For this review, take the finished solid that the model builds, in its own axes (mm). Coordinates: 2 decimals unless noted, no trailing zeros. Write each loop counter-clockwise with the first axis right and the second up, starting at its lowest first coordinate (ties: lowest second). Pieces come first, ordered by that corner, then holes. Notation, with made-up numbers: M 29.25,-34 L 36.25,-34 A25 ccw 36.25,-11 Z; hole C 12.25,53.25 d4. An arc over 180 degrees is marked long. Return JSON: item names as keys, results as strings.
```python
from build123d import *

# Parameters (mm, degrees)
THREAD1_PITCH = 2


with BuildPart() as part:
    # Sketch1 → Revolve3 (revolve)
    with BuildSketch(Plane.XY):
        with BuildLine():
            Line((-5, 97.371710471), (-5, 94.868329805))
            ThreePointArc((-5, 94.868329805), (65.383484153, 68.92024376), (95, 0))
            Line((95, 0), (100, 0))
            ThreePointArc((100, 0), (72.456883731, 68.92024376), (5, 99.874921777))
            Line((5, 99.874921777), (5, 97.371710471))
            Line((5, 97.371710471), (-5, 97.371710471))
        make_face()
    revolve(axis=Axis((-5, 0, 0), (1, 0, 0)))

    # Thread1: arcs per turn and ends read off the stored shape
    # Thread1: the profile of Thread Profile2 profile screwed along a right-hand helix through 5 turns, 10 arcs to a turn; built about Z, then put on its axis
    thread1_z = Axis((0, 0, 0), (0, 0, 1))
    thread1_corners = [(97.371410471, 0, -0.000173205), (98.454242221, 0, 0.624999997), (98.454242221, 0, 0.874999997), (97.371410471, 0, 1.5001732)]
    with BuildLine(mode=Mode.PRIVATE) as thread1_profile:
        Line(thread1_corners[0], thread1_corners[1])
        Line(thread1_corners[1], thread1_corners[2])
        Line(thread1_corners[2], thread1_corners[3])
        Line(thread1_corners[3], thread1_corners[0])
    thread1_cap = Face(thread1_profile.wire())
    thread1_turn_angles = [0, 18, 36, 54, 72, 90, 108, 126, 144, 162, 180, 198, 216, 234, 252, 270, 288, 306, 324, 342, 360]
    thread1_turn_weights = [1, 0.9510565162951535, 1, 0.9510565162951535, 1, 0.9510565162951535, 1, 0.9510565162951535, 1, 0.9510565162951535, 1, 0.9510565162951535, 1, 0.9510565162951535, 1, 0.9510565162951535, 1, 0.9510565162951535, 1, 0.9510565162951535, 1]
    thread1_turn_rails = [Edge.make_bspline([Vector(p[0], p[1], 0).rotate(thread1_z, thread1_turn_angles[k]) / thread1_turn_weights[k] + Vector(0, 0, p[2] + THREAD1_PITCH * thread1_turn_angles[k] / 360) for k in range(21)], [0, 0, 0, 1, 1, 2, 2, 3, 3, 4, 4, 5, 5, 6, 6, 7, 7, 8, 8, 9, 9, 10, 10, 10], 2, thread1_turn_weights) for p in thread1_corners]
    thread1_turn_sides = [Face.make_surface_from_curves(thread1_turn_rails[p[0]], thread1_turn_rails[p[1]]) for p in [(0, 1), (1, 2), (2, 3), (3, 0)]]
    thread1 = Plane(origin=(-5, 0, 0), x_dir=(0, 0, -1), z_dir=(1, 0, 0)) * Solid(Shell([*[p.moved(Location((0, 0, THREAD1_PITCH * i))) for i in range(5) for p in thread1_turn_sides], thread1_cap, thread1_cap.rotate(thread1_z, 1800).moved(Location((0, 0, THREAD1_PITCH * 1800 / 360)))]))
    add(thread1)


solid = part.part
```
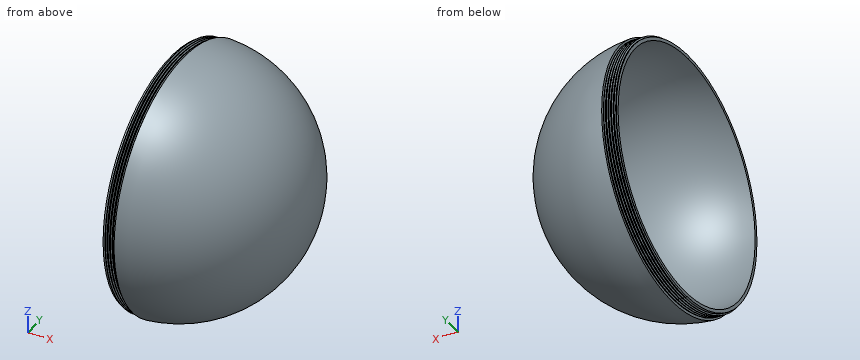
1. We need section A-A (x = 82). State the section outline as (y, z) points.
Checks:
{"outline": "C 0,0 d114.47; hole C 0,0 d95.94"}
2. Wall thickness on L1, parallel to Y at x = 8.5, z = -78.5; L2, parallel to Z at x = 30.5, y = -23; L3, parallel to Z at x = 65, y = 44.5: over which ranges is each line inside the solid? List them lowest first. Write a range as from..to.
Checks:
{"L1": "-61.36..-52.83, 52.83..61.36", "L2": "-92.42..-86.98, 86.98..92.42", "L3": "-61.6..-53.1, 53.1..61.6"}
3. Clearance check with flat-ended pins moving along their axes: pin 1 Ø1 at (x, z) = (88.5, -24) entering from -Y; pin 2 Ø1 at (x, y) = (66.5, -9) entering from +Z; pin 3 Ø1 at (x, z) = (78.5, 22.5) entering from -Y; pin 4 Ø6 at (x, z) = (79, -69.5) entering from -Y. State where each tip first meets the part, or that it passes through.
Checks:
{"pin 1": "y = -41.03", "pin 2": "z = 74.59", "pin 3": "y = -58.42", "pin 4": "through"}
